Verification items for this drawing (mm, ordinates from the low corner). Round coordinates to 2 decimals unless told otherwise and drop trailing zeros. Order: outer loops, then holes, each group sorted by start corner. A loop starts at its lowest first (then second) coordinate and runs counter-clockwise, first axis right, second up. Notation, with made-up numbers: M 11.25,40 L 48.25,40 A19 ccw 48.25,44 Z; hole C -38,51 d9. An arc over 180 degrees is marked long. Use CSV: the item, a comma, the result in double quotes. Start each with the question number.
Q1. Mould release check, pull along X, two halves, no side actions. Record for the marked faces 1 and 2: +X half, -X half, draft (parallel to the pull), parting line (faces both ways), or undercut.
Q2. Sectioned sample at B-B (y = 21.5). Enter the section's corners in (x, z), and give its area (3 significant figures).
Q3. Scan lines: line 1 (Z direction, x = 50, y = 21.5); line 2 (Z direction, x = 37, y = 37); line 3 (X direction, y = 12.5, z = 40.5). Record each from-to range of solid material in increasing order.
Q4. Sectioned sample at C-C (y = 11.5). Enter the section's corners in (x, z).
Q5. Sectioned sample at A-A (z = 50). Enter the section's corners in (x, y), and give its area (3 significant figures).
Q6. Gauge pin test, flat ends, axial feed: pin 1 Ø1.5 at (x, z) = (75, 32.5) entering from +Y; pin 2 Ø2 at (y, z) = (7, 48.5) entering from -X; pin 3 Ø12 at (x, y) = (80.5, 22.5) entering from -Z; pin 4 Ø2 at (x, z) = (68.5, 77) entering from -Y. Record the tip position at first contact, or that the pin passes through.
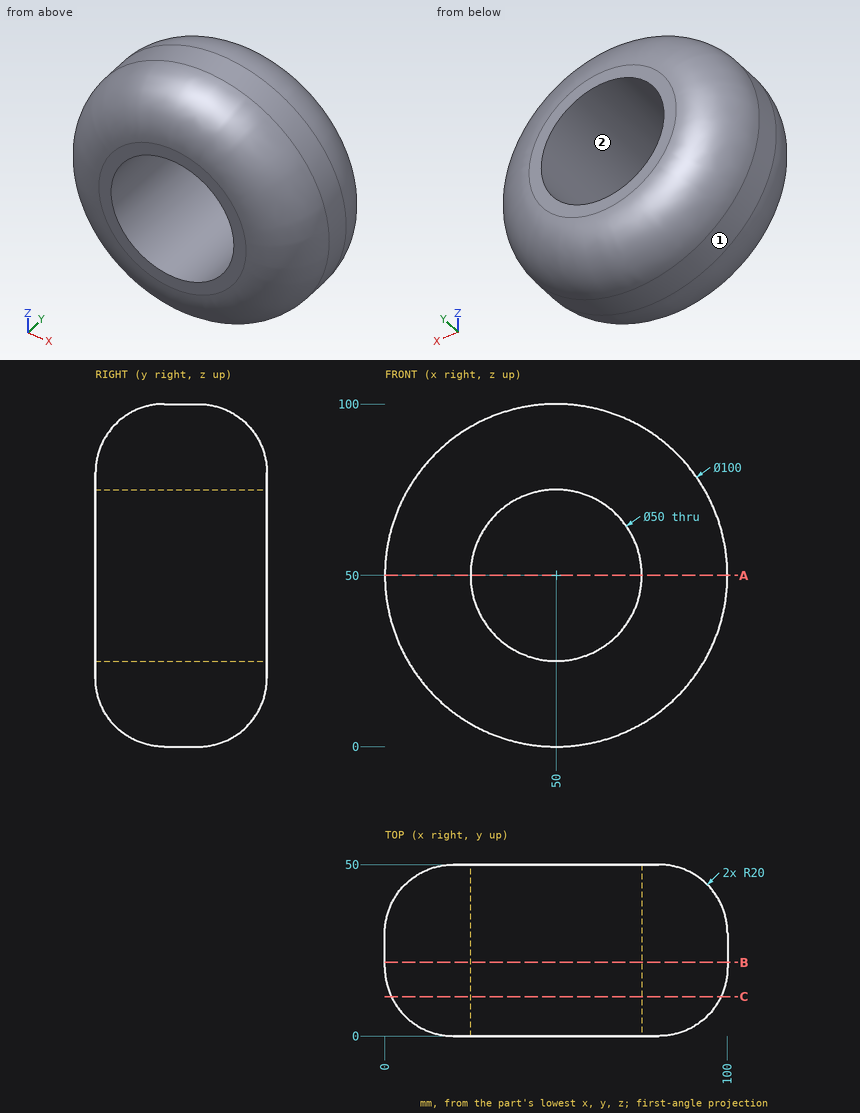
Verdict:
1,face 1,"parting line"
1,face 2,"undercut"
2,outline,"C 50,50 d100; hole C 50,50 d50"
2,area,"5,890 mm²"
3,line 1,"z = 0 to 25, 75 to 100"
3,line 2,"z = 3.03 to 28.65, 71.35 to 96.97"
3,line 3,"x = 2.4 to 26.88, 73.12 to 97.6"
4,outline,"C 50,50 d96.21; hole C 50,50 d50"
5,outline,"M 0,20 A20 ccw 20,0 L 25,0 L 25,50 L 20,50 A20 ccw 0,30 Z; M 75,0 L 80,0 A20 ccw 100,20 L 100,30 A20 ccw 80,50 L 75,50 Z"
5,area,"2,160 mm²"
6,pin 1,"stops at y = 50"
6,pin 2,"stops at x = 4.02"
6,pin 3,"stops at z = 6.41"
6,pin 4,"stops at y = 0.07"
